The drawing under review shows one solid part. Ordinate dimensions are in mm from its lowest x, y, z. A direction names the side the tool comes from. Coordinates: 2 decimals unless noted, no trailing zeros. Order: outer loops, then holes, each group sorted by start corner. A loop starts at its lowest first (then second) coordinate and runs counter-clockwise, first axis right, second up.
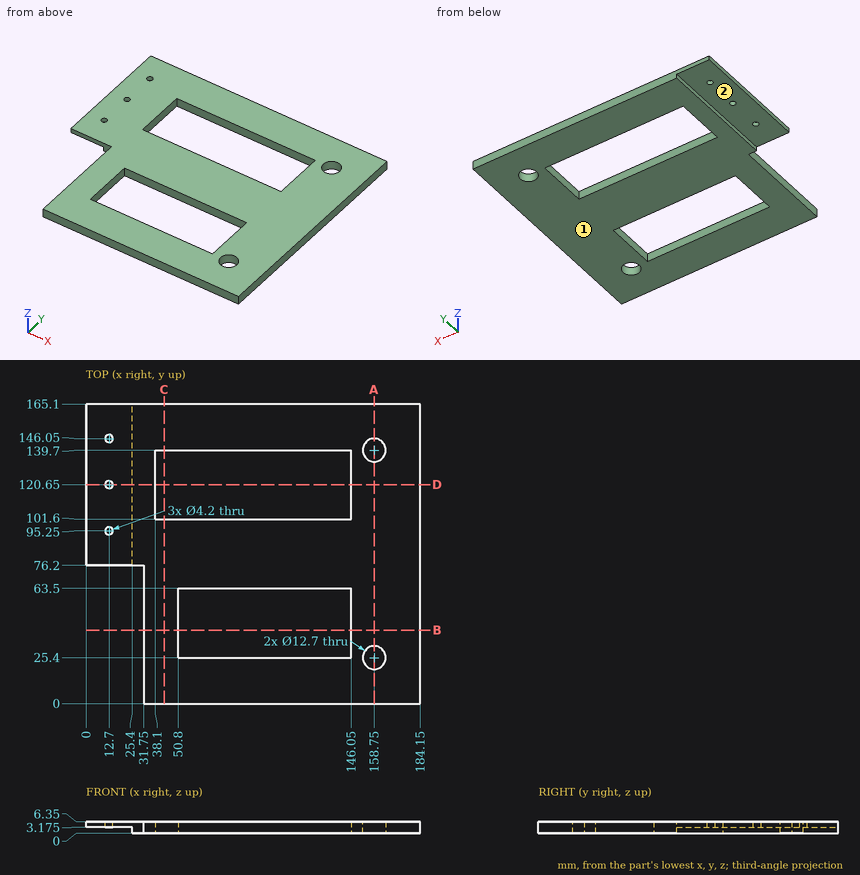
(1) For pin 1 Ø1.9 at (y, z) = (36, 3.5) entering from -X; pin 2 Ø1.9 at (x, z) = (23.5, 2.5) entering from -Y, all flat-tipped, find the tip position at first contact; note any pin that passes through.
A:
pin 1: stops at x = 31.75
pin 2: stops at y = 76.2
(2) Wall thickness on probe 1 along Y at (x, z) = (81, 4); probe 2 along Y at (x, z) = (12.7, 3.9); probe 3 along Y at (x, z) = (158.75, 3.5): over which ranges is each line inside the solid? List them lowest first.
A:
probe 1: y = 0 to 25.4, 63.5 to 101.6, 139.7 to 165.1
probe 2: y = 76.2 to 93.15, 97.35 to 118.55, 122.75 to 143.95, 148.15 to 165.1
probe 3: y = 0 to 19.05, 31.75 to 133.35, 146.05 to 165.1
(3) We need section D-D, the plane y = 120.65. Write out the cut boundary in (x, z) (3 decimals), and give its area (3 significant figures).
A:
outline: (0, 3.175) - (10.6, 3.175) - (10.6, 6.35) - (0, 6.35) - close; (14.8, 3.175) - (25.4, 3.175) - (25.4, 0) - (38.1, 0) - (38.1, 6.35) - (14.8, 6.35) - close; (146.05, 0) - (184.15, 0) - (184.15, 6.35) - (146.05, 6.35) - close
area: 390 mm2
(4) Machinability: for the marked faces 1 and 2, which of the approach directions +Z, -Z, +X, -X, +Y, -Y give a long, thin tool a straight path to every point of the face, cutting with its end or side? Answer none if there is none.
A:
face 1: -Z, +X, -X, +Y, -Y
face 2: -Z, -X, +Y, -Y
(5) We need section C-C, the plane x = 43. Write out the cut boundary in (y, z), and give its area (3 significant figures).
A:
outline: (0, 0) - (101.6, 0) - (101.6, 6.35) - (0, 6.35) - close; (139.7, 0) - (165.1, 0) - (165.1, 6.35) - (139.7, 6.35) - close
area: 806 mm2
(6) We need section B-B, the plane y = 40.5. Write out the cut boundary in (x, z).
A:
outline: (31.75, 0) - (50.8, 0) - (50.8, 6.35) - (31.75, 6.35) - close; (146.05, 0) - (184.15, 0) - (184.15, 6.35) - (146.05, 6.35) - close
(7) We need section A-A, the plane x = 158.75. Write out the cut boundary in (y, z).
A:
outline: (0, 0) - (19.05, 0) - (19.05, 6.35) - (0, 6.35) - close; (31.75, 0) - (133.35, 0) - (133.35, 6.35) - (31.75, 6.35) - close; (146.05, 0) - (165.1, 0) - (165.1, 6.35) - (146.05, 6.35) - close
